The listing builds one solid part. Answer for the finished solid, in the listing's coordinates (mm). A direction names the side the tool comes from. Coordinates: 2 decimals unless noted, no trailing zeros. Write each loop counter-clockwise with the first axis right and the second up, starting at its lowest first coordinate (ties: lowest second). Pieces come first, ordered by that corner, then holes.
(1) The part is cut by section C-C on z = 4.25. Give the number of separate pieces and of enclosed holes in the cut face, plus the area to 3 significant figures.
(2) The part is cut by section D-D on y = 6. Determine the outline of the cut face in (x, z), plus the area to 3 significant figures.
(3) Which of the six approach directions +Z, -Z, +X, -X, +Y, -Y give full straight-line access (tool end or side, diameter ignored) to faces 4 (the cylindrical face through (22.264, 8.737, 0.084)), 5 (the flat face through (59.985, 91, 0))?
(4) The part is cut by section A-A on y = 67. Determine the outline of the cut face in (x, z).
(5) For a pull along Y with two mould halves and no side action, classify faces 1 (the cylindrical face through (49.73, 58.7, -0.08)), 2 (the flat face through (-17.62, 23.78, 0.08)), 3 (the flat face through (20, 55, 6)) as +Y half, -Y half, draft (parallel to the pull), parting line (faces both ways), or undercut.
(6) Straight lines are drawn through the part: line 1 (X direction, y = 59.5, z = -5); line 2 (Y direction, x = -21, z = 1.25); line 3 (Y direction, x = 49.5, z = 5.5). For each, find the intervals that lie inside material, in ascending order.
(7) The part is cut by section B-B on x = 7.5. Determine the outline of the cut face in (y, z), plus the area to 3 significant figures.
(8) Given P1, Ø4, axis at y = 57.5, z = -3.5, coming from the +X side; P2, Ø1.5, axis at x = -24.5, z = 4, coming from the -Y side, each flat-ended and moving along its own axis, determine where each tip first touches the part or whether it passes through.
from build123d import *

# Parameters (mm, degrees)
SKETCH1_R           = 30.75
SKETCH1_R_2         = 3.325
BOSS_EXTRUDE1_DEPTH = 6
SKETCH2_R           = 4.05
CUT_EXTRUDE1_DEPTH  = 161.436981194
LPATTERN1_COUNT     = 3
LPATTERN1_PITCH     = 23


with BuildPart() as part:
    # Sketch1 → Boss-Extrude1 (new, symmetric)
    with BuildSketch(Plane.XY):
        with BuildLine():
            Line((-34.748577527, 46.893721429), (0, 0))
            Line((0, 0), (78.24898238, 0))
            Line((78.24898238, 0), (78.24898238, 15))
            Line((78.24898238, 15), (61.096720235, 48.264425218))
            ThreePointArc((61.096720235, 48.264425218), (60.266695593, 50.489412932), (59.984720032, 52.847378372))
            Line((59.984720032, 52.847378372), (59.984720032, 129.546127467))
            ThreePointArc((59.984720032, 129.546127467), (57.055787843, 136.617195279), (49.984720032, 139.546127467))
            Line((49.984720032, 139.546127467), (-26.714029064, 139.546127467))
            ThreePointArc((-26.714029064, 139.546127467), (-33.785096876, 136.617195279), (-36.714029064, 129.546127467))
            Line((-36.714029064, 129.546127467), (-36.714029064, 52.847378372))
            ThreePointArc((-36.714029064, 52.847378372), (-36.209961999, 49.712532653), (-34.748577527, 46.893721429))
        make_face()
        with Locations((11.87148929, 94.76591255)):
            Circle(SKETCH1_R, mode=Mode.SUBTRACT)
        with Locations((46.66148929, 129.55591255)):
            Circle(SKETCH1_R_2, mode=Mode.SUBTRACT)
        with Locations((46.66148929, 59.97591255)):
            Circle(SKETCH1_R_2, mode=Mode.SUBTRACT)
        with Locations((-22.91851071, 59.97591255)):
            Circle(SKETCH1_R_2, mode=Mode.SUBTRACT)
        with Locations((-22.91851071, 129.55591255)):
            Circle(SKETCH1_R_2, mode=Mode.SUBTRACT)
    extrude(amount=BOSS_EXTRUDE1_DEPTH, both=True)

    # Sketch2 → Cut-Extrude1 (cut, through all)
    with BuildSketch(Plane.XY.offset(6)):
        with Locations((71.24898238, 6)):
            Circle(SKETCH2_R)
    cut_extrude1 = extrude(amount=-CUT_EXTRUDE1_DEPTH, mode=Mode.SUBTRACT)

    # LPattern1: Cut-Extrude1 ×3
    with Locations(*[(-i * LPATTERN1_PITCH, 0, 0) for i in range(1, LPATTERN1_COUNT)]):
        add(cut_extrude1, mode=Mode.SUBTRACT)


solid = part.part
Model answer:
1. separate pieces: 1
1. enclosed holes: 8
1. area: 9,870 mm2
2. outline: (-4.45, -6) - (21.2, -6) - (21.2, 6) - (-4.45, 6) - close; (29.3, -6) - (44.2, -6) - (44.2, 6) - (29.3, 6) - close; (52.3, -6) - (67.2, -6) - (67.2, 6) - (52.3, 6) - close; (75.3, -6) - (78.25, -6) - (78.25, 6) - (75.3, 6) - close
2. area: 701 mm2
3. face 4: +Z, -Z
3. face 5: +Z, -Z, +X, +Y
4. outline: (-36.71, -6) - (-1.34, -6) - (-1.34, 6) - (-36.71, 6) - close; (25.09, -6) - (59.98, -6) - (59.98, 6) - (25.09, 6) - close
5. face 1: undercut
5. face 2: -Y half
5. face 3: draft
6. line 1: x = -36.71 to -26.21, -19.63 to 43.37, 49.95 to 59.98
6. line 2: y = 28.34 to 57.26, 62.69 to 126.84, 132.27 to 139.55
6. line 3: y = 0 to 2.15, 9.85 to 58.24, 61.71 to 127.82, 131.29 to 139.55
7. outline: (0, -6) - (64.33, -6) - (64.33, 6) - (0, 6) - close; (125.2, -6) - (139.55, -6) - (139.55, 6) - (125.2, 6) - close
7. area: 944 mm2
8. P1: stops at x = 59.98
8. P2: stops at y = 32.05
